Read the model definition and answer for the solid it produces. Units are mm, in the model's axes. A direction names the side the tool comes from. Coordinates: 2 decimals unless noted, no trailing zeros. Loops run counter-clockwise (first coordinate to the right, second up) from the corner with the lowest first, then second, coordinate; pieces in that order, holes last. Notation, with made-up numbers: (-14, 58) -> (42, 58) arc R22 cw to (42, 84) -> close; hole circle Ø2 at (34, 68). An arc over 180 degrees is marked (long way). Answer as a JSON object with one key per item and string values. Group by question number.
1) Section B-B, the plane y = 12.25 is taken. Give the vertices of the cut face in (x, z), plus the area to 3 significant figures.
2) Section D-D, the plane y = 21 is taken. Give the vertices of the cut face in (x, z).
3) Flat-ended cylindrical pins translate along their axes: P1, Ø8, axis at x = 22, z = -28.5, coming from the +Y side; P2, Ø4.5, axis at x = 23.69, y = 5, coming from the -Z side; P3, Ø3, axis at y = 5, z = 7.1, coming from the -X side. Find the tip coordinate at first contact, or state that the pin passes through.
4) Determine the mould class of faces 1 (the face through (15.53, 6.69, -36.91)), 2 (the face through (-19.3, 5.1, 4.6)), 3 (the face through (-19.33, 6.69, -14.74)) for opening direction Z: released by +Z, released by -Z, zero draft, split by the parting line, or undercut.
5) Section A-A, the plane z = 7.1 is taken. Give the vertices of the cut face in (x, y), plus the area to 3 significant figures.
6) Consider probe 1 along X at (y, z) = (11.5, -17.5); probe 2 along Z at (x, y) = (18.5, 6); probe 3 along Y at (x, z) = (36.4, -32.9). Determine where each line is inside the solid, lowest interval first. Write a range as [from, to].
7) Which of the six approach directions +Z, -Z, +X, -X, +Y, -Y give full straight-line access (tool end or side, diameter ignored) to faces 4 (the face through (8, 13, -35.9)), 5 (the face through (4.01, 7.48, -36.91)), 6 (the face through (32.386, 9, 31))?
8) Section C-C, the plane x = -12 is taken. Give the vertices of the cut face in (y, z), plus the area to 3 significant figures.
Autodesk Inventor part; units mm, degrees
ref_plane "YZ Plane" through (0, 0, 0) normal (1, 0, 0) x (0, 1, 0)
ref_plane "XZ Plane" through (0, 0, 0) normal (0, 1, 0) x (-1, 0, 0)
ref_plane "XY Plane" through (0, 0, 0) normal (0, 0, 1) x (1, 0, 0)
sketch "Sketch1" plane through (0, 0, 0) normal (0, 1, 0) x (-1, 0, 0)
  point P0 (0, 0)
sketch "Sketch2" plane through (0, 0, 0) normal (0, 1, 0) x (-1, 0, 0)
  point P0 (0, 0)
sketch "Sketch3" plane through (0, 0, 0) normal (0, 1, 0) x (-1, 0, 0)
  line L0 (20.3143, 32.1) -> (-37.6857, 32.1)
  line L1 (-37.6857, 32.1) -> (-37.6857, -37.9)
  line L2 (-37.6857, -37.9) -> (20.3143, -37.9)
  line L3 (20.3143, -37.9) -> (20.3143, 32.1)
  point P0 (0, 0)
  dimension "d0" = 70
  dimension "d1" = 58
extrude "Extrusion1" add sketch "Sketch3" along normal blind 24
sketch "Sketch4" plane through (0, 24, 0) normal (0, 1, 0) x (1, 0, 0)
  point P0 (0, 0)
sketch "Sketch5" plane through (0, 24, 0) normal (0, 1, 0) x (1, 0, 0)
  line L0 (-18.3143, 35.9) -> (35.6857, 35.9)
  line L1 (35.6857, 35.9) -> (35.6857, -30.1)
  line L2 (35.6857, -30.1) -> (-18.3143, -30.1)
  line L3 (-18.3143, -30.1) -> (-18.3143, 35.9)
  line L4 (37.6857, -32.1) -> (37.6857, 37.9)
  line L5 (-20.3143, -32.1) -> (37.6857, -32.1)
  line L6 (-20.3143, 37.9) -> (-20.3143, -32.1)
  line L7 (37.6857, 37.9) -> (-20.3143, 37.9)
  point P0 (0, 0)
  dimension "d4" = 2
  dimension "d5" = 2
  dimension "d6" = 2
  dimension "d7" = 2
extrude "Extrusion2" cut sketch "Sketch5" against normal blind 22 contours L0 L1 L2 L3
sketch "Sketch6" plane through (-20.3143, 0, 32.1) normal (0, 0, 1) x (1, 0, 0)
  line L0 (9.8, 13.3) -> (21.8, 13.3)
  line L1 (21.8, 13.3) -> (21.8, 3.3)
  line L2 (21.8, 3.3) -> (9.8, 3.3)
  line L3 (9.8, 3.3) -> (9.8, 13.3)
  line L4 (0, 0) -> (0, 24)
  line L5 (0, 0) -> (58, 0)
  point P0 (20.3143, 0)
  dimension "d10" = 9.8
  dimension "d11" = 12
  dimension "d12" = 10
  dimension "d13" = 3.3
extrude "Extrusion3" cut sketch "Sketch6" against normal blind 22.45
sketch "Sketch7" plane through (-20.3143, 0, 32.1) normal (0, 0, 1) x (1, 0, 0)
  line L0 (43.7, 14.2) -> (52.7, 14.2)
  line L1 (52.7, 14.2) -> (52.7, 3.3)
  line L2 (52.7, 3.3) -> (43.7, 3.3)
  line L3 (43.7, 3.3) -> (43.7, 14.2)
  line L4 (58, 0) -> (58, 24)
  line L5 (0, 0) -> (58, 0)
  point P0 (20.3143, 0)
  dimension "d16" = 5.3
  dimension "d17" = 9
  dimension "d18" = 10.9
  dimension "d19" = 3.3
extrude "Extrusion4" cut sketch "Sketch7" against normal blind 25.175
sketch "Sketch8" plane through (-20.3143, 0, -37.9) normal (-1, 0, 0) x (0, 0, 1)
  circle A0 centre (65, 5) radius 2.5
  line L0 (0, 0) -> (70, 0)
  line L1 (70, 0) -> (70, 24)
  circle A1 centre (55, 5) radius 2.5
  circle A2 centre (45, 5) radius 2.5
  circle A3 centre (35, 5) radius 2.5
  circle A4 centre (25, 5) radius 2.5
  circle A5 centre (15, 5) radius 2.5
  circle A6 centre (5, 5) radius 2.5
  point P0 (37.9, 0)
  point P1 (35, 0)
  dimension "d22" = 5
  dimension "d23" = 5
  dimension "d24" = 5
  dimension "d25" = 5
  dimension "d26" = 10
  dimension "d27" = 5
  dimension "d28" = 5
  dimension "d29" = 5
  dimension "d30" = 10
  dimension "d31" = 5
  dimension "d32" = 10
  dimension "d33" = 5
  dimension "d34" = 5
  dimension "d35" = 10
  dimension "d36" = 5
  dimension "d37" = 5
  dimension "d38" = 5
  dimension "d39" = 10
  dimension "d40" = 5
  dimension "d41" = 10
  dimension "d42" = 5
extrude "Extrusion5" cut sketch "Sketch8" against normal blind 44.225
sketch "Sketch9" plane through (-20.3143, 0, -37.9) normal (-1, 0, 0) x (0, 0, 1)
  point P0 (37.9, 0)
sketch "Sketch10" plane through (37.6857, 0, 32.1) normal (1, 0, 0) x (0, 0, -1)
  circle A0 centre (5, 5.0214) radius 2.5
  line L0 (0, 0) -> (0, 24)
  circle A1 centre (15, 5) radius 2.5
  line L1 (0, 0) -> (70, 0)
  circle A2 centre (25, 5) radius 2.5
  circle A3 centre (35, 5) radius 2.5
  circle A4 centre (45, 5) radius 2.5
  circle A5 centre (55, 5) radius 2.5
  circle A6 centre (65, 5) radius 2.5
  point P0 (32.1, 0)
  dimension "d45" = 5
  dimension "d46" = 5
  dimension "d47" = 5
  dimension "d48" = 10
  dimension "d49" = 5
  dimension "d50" = 5
  dimension "d51" = 5
  dimension "d52" = 10
  dimension "d53" = 5
  dimension "d54" = 5
  dimension "d55" = 10
  dimension "d56" = 5
  dimension "d57" = 10
  dimension "d58" = 5
  dimension "d59" = 5
  dimension "d60" = 5
  dimension "d61" = 10
  dimension "d62" = 5
  dimension "d63" = 10
  dimension "d64" = 5
extrude "Extrusion6" cut sketch "Sketch10" against normal blind 41.5
sketch "Sketch11" plane through (37.6857, 0, -37.9) normal (0, 0, -1) x (-1, 0, 0)
  circle A0 centre (4, 5) radius 2.5
  line L0 (0, 0) -> (0, 24)
  line L1 (0, 0) -> (58, 0)
  circle A1 centre (14, 5) radius 2.5
  circle A2 centre (24, 5) radius 2.5
  circle A3 centre (34, 5) radius 2.5
  circle A4 centre (44, 5) radius 2.5
  circle A5 centre (54, 5) radius 2.5
  point P0 (37.6857, 0)
  dimension "d67" = 5
  dimension "d68" = 4
  dimension "d69" = 5
  dimension "d70" = 5
  dimension "d71" = 10
  dimension "d72" = 5
  dimension "d73" = 5
  dimension "d74" = 10
  dimension "d75" = 5
  dimension "d76" = 5
  dimension "d77" = 10
  dimension "d78" = 5
  dimension "d79" = 5
  dimension "d80" = 10
  dimension "d81" = 5
  dimension "d82" = 5
  dimension "d83" = 10
  dimension "d84" = 5
extrude "Extrusion7" cut sketch "Sketch11" against normal blind 2
properties part number "junction box"
Determined:
{
 "1": {"outline": "(-20.31, -37.9) -> (37.69, -37.9) -> (37.69, 32.1) -> (32.39, 32.1) -> (32.39, 30.1) -> (35.69, 30.1) -> (35.69, -35.9) -> (-18.31, -35.9) -> (-18.31, 30.1) -> (-10.51, 30.1) -> (-10.51, 32.1) -> (-20.31, 32.1) -> close; (1.49, 30.1) -> (23.39, 30.1) -> (23.39, 32.1) -> (1.49, 32.1) -> close", "area": "454 mm²"},
 "2": {"outline": "(-20.31, -37.9) -> (37.69, -37.9) -> (37.69, 32.1) -> (-20.31, 32.1) -> close; hole (-18.31, -35.9) -> (35.69, -35.9) -> (35.69, 30.1) -> (-18.31, 30.1) -> close"},
 "3": {"P1": "y = 2", "P2": "z = 30.1", "P3": "through"},
 "4": {"face 1": "zero draft", "face 2": "undercut", "face 3": "undercut"},
 "5": {"outline": "(-20.31, 0) -> (37.69, 0) -> (37.69, 2.5) -> (35.69, 2.5) -> (35.69, 2) -> (-18.31, 2) -> (-18.31, 2.5) -> (-20.31, 2.5) -> close; (-20.31, 7.5) -> (-18.31, 7.5) -> (-18.31, 24) -> (-20.31, 24) -> close; (35.69, 7.5) -> (37.69, 7.5) -> (37.69, 24) -> (35.69, 24) -> close", "area": "184 mm²"},
 "6": {"probe 1": "[-20.31, -18.31], [35.69, 37.69]", "probe 2": "[-37.9, -35.9], [30.1, 32.1]", "probe 3": "[0, 2.5], [7.5, 24]"},
 "7": {"face 4": "+Y", "face 5": "-Z", "face 6": "+Z"},
 "8": {"outline": "(0, -37.9) -> (24, -37.9) -> (24, -35.9) -> (2, -35.9) -> (2, 30.1) -> (24, 30.1) -> (24, 32.1) -> (0, 32.1) -> close", "area": "228 mm²"}
}
